from build123d import *

# Parameters (mm, degrees)
SKETCH1_W                                  = 170
SKETCH1_H                                  = 150
BOSS_EXTRUDE1_DEPTH                        = 10
BOSS_EXTRUDE2_DEPTH                        = 170
FILLET1_R                                  = 10
SHELL1_T                                   = -2
SKETCH3_W                                  = 115
SKETCH3_H                                  = 90
CUT_EXTRUDE1_DEPTH                         = 2
SKETCH4_W                                  = 119
SKETCH4_H                                  = 94
SKETCH4_W_2                                = 115
SKETCH4_H_2                                = 90
BOSS_EXTRUDE3_DEPTH                        = 10
SKETCH5_W                                  = 119
SKETCH5_H                                  = 94
BOSS_EXTRUDE4_DEPTH                        = 2
SKETCH6_R                                  = 2.5
CUT_EXTRUDE2_DEPTH                         = 2
SKETCH7_R                                  = 6
CUT_EXTRUDE3_DEPTH                         = 2
SKETCH9_W                                  = 10
SKETCH9_H                                  = 15
BOSS_EXTRUDE5_DEPTH                        = 10
SKETCH10_W                                 = 5
SKETCH10_H                                 = 10
CUT_EXTRUDE4_DEPTH                         = 5
MIRROR1_AT_THE_SECOND_PLANE_COPY_1_SKETC_W = 10
MIRROR1_AT_THE_SECOND_PLANE_COPY_1_SKETC_H = 15
MIRROR1_AT_THE_SECOND_PLANE_COPY_1_DEPTH   = 10
MIRROR1_AT_THE_SECOND_PLANE_COPY_2_SKETC_W = 5
MIRROR1_AT_THE_SECOND_PLANE_COPY_2_SKETC_H = 10
MIRROR1_AT_THE_SECOND_PLANE_COPY_2_DEPTH   = 5
FILLET2_R                                  = 2


with BuildPart() as part:
    # Sketch1 → Boss-Extrude1 (new body)
    with BuildSketch(Plane(origin=(0, 0, 0), x_dir=(1, 0, 0), z_dir=(0, 1, 0))):
        Rectangle(SKETCH1_W, SKETCH1_H)
    extrude(amount=BOSS_EXTRUDE1_DEPTH)

    # Sketch2 → Boss-Extrude2 (add)
    with BuildSketch(Plane.ZY.offset(85)):
        Polygon((-75, 10), (-75, 50.192378865), (75, 10), align=None)
    extrude(amount=-BOSS_EXTRUDE2_DEPTH)

    # Fillet1
    fillet1_edges = [part.edges().sort_by_distance(p)[0] for p in [
        (0, 50.192378865, -75),
        (-85, 30.096189432, 0),
        (85, 30.096189432, 0),
        (0, 10, 75),
        (85, 5, 75),
        (-85, 5, 75),
        (-85, 25.096189432, -75),
        (85, 25.096189432, -75),
    ]]
    fillet(fillet1_edges, radius=FILLET1_R)

    # Shell1
    shell1_openings = [part.faces().sort_by_distance(p)[0] for p in [
        (0, 0, 0),
    ]]
    offset(amount=SHELL1_T, openings=shell1_openings, kind=Kind.INTERSECTION)

    # Sketch3 → Cut-Extrude1 (cut)
    with BuildSketch(Plane(origin=(0, 28.080127019, 7.524047358), x_dir=(1, 0, 0), z_dir=(0, 0.96592582628907, 0.25881904510251436))):
        with Locations((0, 10)):
            Rectangle(SKETCH3_W, SKETCH3_H)
    extrude(amount=-CUT_EXTRUDE1_DEPTH, mode=Mode.SUBTRACT)

    # Sketch4 → Boss-Extrude3 (add)
    with BuildSketch(Plane(origin=(0, 26.148275366, 7.006409268), x_dir=(1, 0, 0), z_dir=(0, -0.96592582628907, -0.25881904510251436))):
        with Locations((0, -10)):
            Rectangle(SKETCH4_W, SKETCH4_H)
        with Locations((0, -10)):
            Rectangle(SKETCH4_W_2, SKETCH4_H_2, mode=Mode.SUBTRACT)
    extrude(amount=BOSS_EXTRUDE3_DEPTH)

    # Sketch5 → Boss-Extrude4 (add)
    with BuildSketch(Plane(origin=(0, 16.489017103, 4.418218817), x_dir=(1, 0, 0), z_dir=(0, -0.96592582628907, -0.25881904510251436))):
        with Locations((0, -10)):
            Rectangle(SKETCH5_W, SKETCH5_H)
    extrude(amount=BOSS_EXTRUDE4_DEPTH)

    # Sketch6 → Cut-Extrude2 (cut)
    with BuildSketch(Plane(origin=(0, 28.080127019, 7.524047358), x_dir=(1, 0, 0), z_dir=(0, 0.96592582628907, 0.25881904510251436))):
        with Locations(Location((-62.5, 10, 0), (0, 0, 270))):
            Circle(SKETCH6_R)
        with Locations(Location((-62.5, 40, 0), (0, 0, 270))):
            Circle(SKETCH6_R)
        with Locations(Location((-62.5, -20, 0), (0, 0, 270))):
            Circle(SKETCH6_R)
        with Locations(Location((62.5, -20, 0), (0, 0, 270))):
            Circle(SKETCH6_R)
        with Locations(Location((62.5, 40, 0), (0, 0, 270))):
            Circle(SKETCH6_R)
        with Locations(Location((62.5, 10, 0), (0, 0, 270))):
            Circle(SKETCH6_R)
    extrude(amount=-CUT_EXTRUDE2_DEPTH, mode=Mode.SUBTRACT)

    # Sketch7 → Cut-Extrude3 (cut)
    with BuildSketch(Plane(origin=(0, 28.080127019, 7.524047358), x_dir=(1, 0, 0), z_dir=(0, 0.96592582628907, 0.25881904510251436))):
        with Locations(Location((-12.5, -48.59148832, 0), (0, 0, 270))):
            Circle(SKETCH7_R)
        with Locations(Location((12.5, -48.59148832, 0), (0, 0, 270))):
            Circle(SKETCH7_R)
        with Locations(Location((37.5, -48.59148832, 0), (0, 0, 270))):
            Circle(SKETCH7_R)
        with Locations(Location((-37.5, -48.59148832, 0), (0, 0, 270))):
            Circle(SKETCH7_R)
    extrude(amount=-CUT_EXTRUDE3_DEPTH, mode=Mode.SUBTRACT)

    # Sketch9 → Boss-Extrude5 (add)
    with BuildSketch(Plane.XZ):
        with Locations((-78, -47.5)):
            Rectangle(SKETCH9_W, SKETCH9_H)
    boss_extrude5 = extrude(amount=-BOSS_EXTRUDE5_DEPTH)

    # Sketch10 → Cut-Extrude4 (cut)
    with BuildSketch(Plane.XZ):
        with Locations((-78, -47.5)):
            Rectangle(SKETCH10_W, SKETCH10_H)
    cut_extrude4 = extrude(amount=-CUT_EXTRUDE4_DEPTH, mode=Mode.SUBTRACT)

    # Mirror1: Boss-Extrude5, Cut-Extrude4 across plane
    add(boss_extrude5.mirror(Plane(origin=(0, 0, 0), x_dir=(0, 0, 1), z_dir=(1, 0, 0))))
    add(cut_extrude4.mirror(Plane(origin=(0, 0, 0), x_dir=(0, 0, 1), z_dir=(1, 0, 0))), mode=Mode.SUBTRACT)

    # Mirror1 at the second plane: Boss-Extrude5, Cut-Extrude4 across plane
    add(boss_extrude5.mirror(Plane.XY))
    add(cut_extrude4.mirror(Plane.XY), mode=Mode.SUBTRACT)

    # Mirror1 at the second plane copy 1 sketc → Mirror1 at the second plane copy 1 (add)
    with BuildSketch(Plane(origin=(0, 0, 0), x_dir=(-1, 0, 0), z_dir=(0, -1, 0))):
        with Locations((-78, -47.5)):
            Rectangle(MIRROR1_AT_THE_SECOND_PLANE_COPY_1_SKETC_W, MIRROR1_AT_THE_SECOND_PLANE_COPY_1_SKETC_H)
    extrude(amount=-MIRROR1_AT_THE_SECOND_PLANE_COPY_1_DEPTH)

    # Mirror1 at the second plane copy 2 sketc → Mirror1 at the second plane copy 2 (cut)
    with BuildSketch(Plane(origin=(0, 0, 0), x_dir=(-1, 0, 0), z_dir=(0, -1, 0))):
        with Locations((-78, -47.5)):
            Rectangle(MIRROR1_AT_THE_SECOND_PLANE_COPY_2_SKETC_W, MIRROR1_AT_THE_SECOND_PLANE_COPY_2_SKETC_H)
    extrude(amount=-MIRROR1_AT_THE_SECOND_PLANE_COPY_2_DEPTH, mode=Mode.SUBTRACT)

    # Fillet2
    fillet2_edges = [part.edges().sort_by_distance(p)[0] for p in [
        (-73, 5, -40),
        (-73, 5, -55),
        (-73, 5, 40),
        (-73, 5, 55),
        (73, 5, -55),
        (73, 5, -40),
        (73, 5, 55),
        (73, 5, 40),
    ]]
    fillet(fillet2_edges, radius=FILLET2_R)


solid = part.part
The listing builds one solid part. Answer for the finished solid, in the listing's coordinates (mm). A direction names the side the tool comes from. Round coordinates to 2 decimals unless told otherwise and drop trailing zeros. Order: outer loops, then holes, each group sorted by start corner. A loop starts at its lowest first (then second) coordinate and runs counter-clockwise, first axis right, second up. Notation, with made-up numbers: (86, -9.5) - (93, -9.5) arc R21 ccw to (93, 24.5) - close; hole circle Ø3 at (60, -7). An arc over 180 degrees is marked (long way). Write item = value, one per line. Start each with the question number.
1) Straight lines are drawn through the part: L1, parallel to X at y = 14, z = -44; L2, parallel to Z at x = 59.5, y = 3.5; L3, parallel to X at y = 22.5, z = 22. For each, find the intervals that lie inside material, in ascending order.
2) For faces 1 (the flat face through (-83, 15, -23)), 2 (the flat face through (-79, 5, -40)), determine the directions among +Z, -Z, +X, -X, +Y, -Y from which every point of the face is accessible in a straight line to the end or side of a thin tool.
3) Section A-A, the plane x = 67 is taken. Write down the section's boundary in (y, z), plus the area to 3 significant figures.
4) For a pull along Z with two mould halves and no side action, classify faces 3 (the cylindrical face through (1.05, 8.34, 72.99)), 4 (the cylindrical face through (81.99, 18.32, -72.15)), 5 (the flat face through (-79, 5, 55)) as released by +Z, released by -Z, zero draft, split by the parting line, or undercut.
5) Section C-C, the plane x = -46 is taken. Write down the section's boundary in (y, z), plus the area to 3 significant figures.
6) Section B-B, the plane z = -32 is taken. Count the separate pieces of the cut face and the enclosed holes in it, plus the area to 3 significant figures.
7) Given pin 1 (11 mm diameter, centred on x = -78.5, z = 49, fed in from +Y); pin 2 (1.5 mm diameter, centred on x = 77.5, y = 1.5, fed in from -Z); pin 3 (2.5 mm diameter, centred on x = -78.5, z = -49.5, fed in from -Y), each flat-ended and moving along its own axis, determine where each tip first touches the part or whether it passes through.
Results list:
q1.L1 = -85 to -83, 83 to 85
q1.L2 = -75 to -73, 72.91 to 74.93
q1.L3 = -80.49 to -57.5, 57.5 to 80.49
q2.face_1 = none
q2.face_2 = -Y
q3.outline = (0, -75) - (37.16, -75) arc R10 ccw to (46.82, -62.41) - (11.99, 67.59) arc R10 ccw to (2.33, 75) - (0, 75) - (0, 73) - (2.33, 73) arc R8 cw to (10.05, 67.07) - (44.89, -62.93) arc R8 cw to (37.16, -73) - (0, -73) - close
q3.area = 405 mm^2
q4.face_3 = released by +Z
q4.face_4 = released by -Z
q4.face_5 = undercut
q5.outline = (0, -75) - (37.16, -75) arc R10 ccw to (46.82, -62.41) - (42.32, -45.6) - (30.72, -48.71) - (7.43, 38.23) - (19.02, 41.33) - (11.99, 67.59) arc R10 ccw to (2.33, 75) - (0, 75) - (0, 73) - (2.33, 73) arc R8 cw to (10.05, 67.07) - (16.57, 42.75) - (4.98, 39.64) - (29.31, -51.16) - (40.9, -48.05) - (44.89, -62.93) arc R8 cw to (37.16, -73) - (0, -73) - close
q5.area = 453 mm^2
q6.separate_pieces = 3
q6.enclosed_holes = 0
q6.area = 512 mm^2
q7.pin_1 = 18.23
q7.pin_2 = -74.85
q7.pin_3 = 5
